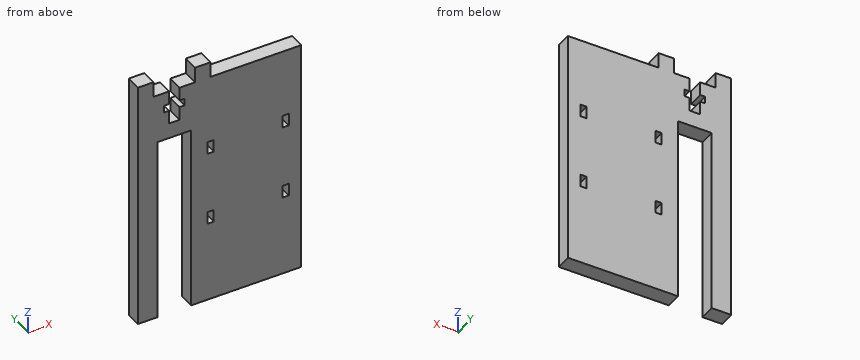
from build123d import *

# Parameters (mm, degrees)
SKETCH1_W           = 2.54
SKETCH1_H           = 5.08
BOSS_EXTRUDE1_DEPTH = 6.35


with BuildPart() as part:
    # Sketch1 → Boss-Extrude1 (new body)
    with BuildSketch(Plane(origin=(0, 0, 0), x_dir=(1, 0, 0), z_dir=(0, 1, 0))):
        Polygon((-6.858, 6.35), (-6.858, 82.55), (-14.859, 82.55), (-14.859, -13.97), (-14.859, -20.32), (-8.509, -20.32), (-8.509, -13.97), (-2.159, -13.97), (-2.159, -8.435000021), (-4.199999982, -8.435000021), (-4.199999982, -5.534999979), (-2.159, -5.534999979), (-2.159, 0), (2.159, 0), (2.159, -5.534999979), (4.199999982, -5.534999979), (4.199999982, -8.435000021), (2.159, -8.435000021), (2.159, -13.97), (8.509, -13.97), (8.509, -20.32), (14.859, -20.32), (14.859, -13.97), (45.593, -13.97), (51.943, -13.97), (51.943, 82.55), (45.593, 82.55), (14.859, 82.55), (6.858, 82.55), (6.858, 6.35), align=None)
        with Locations((14.859, 16.51)):
            Rectangle(SKETCH1_W, SKETCH1_H, mode=Mode.SUBTRACT)
        with Locations((45.593, 16.51)):
            Rectangle(SKETCH1_W, SKETCH1_H, mode=Mode.SUBTRACT)
        with Locations((14.859, 46.99)):
            Rectangle(SKETCH1_W, SKETCH1_H, mode=Mode.SUBTRACT)
        with Locations((45.593, 46.99)):
            Rectangle(SKETCH1_W, SKETCH1_H, mode=Mode.SUBTRACT)
    extrude(amount=BOSS_EXTRUDE1_DEPTH)


solid = part.part
Model file for the job. Use its own axes, mm. Give positions to 0.01 mm unless a question says otherwise; leave off trailing zeros. Order: outer loops, then holes, each group sorted by start corner. A loop starts at its lowest first (then second) coordinate and runs counter-clockwise, first axis right, second up. Notation, with made-up numbers: M 33,47 L 86,47 A19 ccw 86,83 Z; hole C 50.5,12 d11. An arc over 180 degrees is marked long. Put each result on its own line as item: value. Start each with the question number.
(1) Band-saw the part on D-D on y = 3.25. Count the separate pieces of the cut face and the enclosed holes in it, then the cut area to 3 significant figures.
(2) Band-saw the part on C-C on x = 30. Give the cut face in (y, z), then the cut area to 3 significant figures.
(3) Drill centre lines: L1, parallel to X at y = 1.5, z = -44.5; L2, parallel to X at y = 2.25, z = -38; L3, parallel to Z at x = 2.5, y = 3.25 (3 decimals). Where is each one in solid material? Low to high. Write a range as [from, to].
(4) Band-saw the part on A-A on z = -73.5. Give the cut face in (x, y), then the cut area to 3 significant figures.
(5) Band-saw the part on B-B on z = -15. Give the cut face in (x, y), then the cut area to 3 significant figures.
(6) Pin check, flat tips, straight feed: pin 1 Ø3.5 at (x, y) = (-0.5, 3) entering from +Z; pin 2 Ø1.6 at (x, y) = (3, 2) entering from -Z. Stop position of each tip, or through.
Results below:
1. separate pieces: 1
1. enclosed holes: 4
1. area: 5,360 mm2
2. outline: M 0,-82.55 L 6.35,-82.55 L 6.35,13.97 L 0,13.97 Z
2. area: 613 mm2
3. L1: x = [-14.86, -6.86], [6.86, 13.59], [16.13, 44.32], [46.86, 51.94]
3. L2: x = [-14.86, -6.86], [6.86, 51.94]
3. L3: z = [-6.35, 5.535], [8.435, 13.97]
4. outline: M -14.86,0 L -6.86,0 L -6.86,6.35 L -14.86,6.35 Z; M 6.86,0 L 51.94,0 L 51.94,6.35 L 6.86,6.35 Z
4. area: 337 mm2
5. outline: M -14.86,0 L -6.86,0 L -6.86,6.35 L -14.86,6.35 Z; M 6.86,0 L 13.59,0 L 13.59,6.35 L 6.86,6.35 Z; M 16.13,0 L 44.32,0 L 44.32,6.35 L 16.13,6.35 Z; M 46.86,0 L 51.94,0 L 51.94,6.35 L 46.86,6.35 Z
5. area: 305 mm2
6. pin 1: stops at z = 13.97
6. pin 2: stops at z = -6.35
